```python
from build123d import *

# Parameters (mm, degrees)
F0_R     = 2.15
F1_DEPTH = 250


# Not quite as in the source:
# - ends of sketch curves that miss each other by under 0.0002 mm in the source are joined


with BuildPart() as f1:
    # F0 (on Top) → F1 (new body)
    with BuildSketch(Plane.XY):
        with BuildLine():
            Line((10, 3.5), (10, 9))
            ThreePointArc((10, 9), (9.7071067812, 9.7071067812), (9, 10))
            Line((9, 10), (3.5, 10))
            ThreePointArc((3.5, 10), (2.7928932188, 9.7071067812), (2.5, 9))
            Line((2.5, 9), (2.5, 8.2))
            Line((2.5, 8.2), (4.9, 8.2))
            ThreePointArc((4.9, 8.2), (5.8238795325, 7.5826834324), (5.6071067812, 6.4928932188))
            Line((5.6071067812, 6.4928932188), (3.057107, 3.942893))
            ThreePointArc((3.057107, 3.942893), (2.7326834324, 3.7261204675), (2.35, 3.65))
            Line((2.35, 3.65), (-2.35, 3.65))
            ThreePointArc((-2.35, 3.65), (-2.7326834324, 3.7261204675), (-3.0571067812, 3.9428932188))
            Line((-3.0571067812, 3.9428932188), (-5.607107, 6.492893))
            ThreePointArc((-5.607107, 6.492893), (-5.8238795325, 7.5826834324), (-4.9, 8.2))
            Line((-4.9, 8.2), (-2.5, 8.2))
            Line((-2.5, 8.2), (-2.5, 9))
            ThreePointArc((-2.5, 9), (-2.7928932188, 9.7071067812), (-3.5, 10))
            Line((-3.5, 10), (-9, 10))
            ThreePointArc((-9, 10), (-9.7071067812, 9.7071067812), (-10, 9))
            Line((-10, 9), (-10, 3.5))
            ThreePointArc((-10, 3.5), (-9.7071067812, 2.7928932188), (-9, 2.5))
            Line((-9, 2.5), (-8.2, 2.5))
            Line((-8.2, 2.5), (-8.2, 4.9))
            ThreePointArc((-8.2, 4.9), (-7.5826834324, 5.8238795325), (-6.4928932188, 5.6071067812))
            Line((-6.4928932188, 5.6071067812), (-3.942893, 3.057107))
            ThreePointArc((-3.942893, 3.057107), (-3.7261204675, 2.7326834324), (-3.65, 2.35))
            Line((-3.65, 2.35), (-3.65, -2.35))
            ThreePointArc((-3.65, -2.35), (-3.7261204675, -2.7326834324), (-3.9428932188, -3.0571067812))
            Line((-3.9428932188, -3.0571067812), (-6.492893, -5.607107))
            ThreePointArc((-6.492893, -5.607107), (-7.5826834324, -5.8238795325), (-8.2, -4.9))
            Line((-8.2, -4.9), (-8.2, -2.5))
            Line((-8.2, -2.5), (-9, -2.5))
            ThreePointArc((-9, -2.5), (-9.7071067812, -2.7928932188), (-10, -3.5))
            Line((-10, -3.5), (-10, -9))
            ThreePointArc((-10, -9), (-9.7071067812, -9.7071067812), (-9, -10))
            Line((-9, -10), (-3.5, -10))
            ThreePointArc((-3.5, -10), (-2.7928932188, -9.7071067812), (-2.5, -9))
            Line((-2.5, -9), (-2.5, -8.2))
            Line((-2.5, -8.2), (-4.9, -8.2))
            ThreePointArc((-4.9, -8.2), (-5.8238795325, -7.5826834324), (-5.6071067812, -6.4928932188))
            Line((-5.6071067812, -6.4928932188), (-3.057107, -3.942893))
            ThreePointArc((-3.057107, -3.942893), (-2.7326834324, -3.7261204675), (-2.35, -3.65))
            Line((-2.35, -3.65), (2.35, -3.65))
            ThreePointArc((2.35, -3.65), (2.7326834324, -3.7261204675), (3.0571067812, -3.9428932188))
            Line((3.0571067812, -3.9428932188), (5.607107, -6.492893))
            ThreePointArc((5.607107, -6.492893), (5.8238795325, -7.5826834324), (4.9, -8.2))
            Line((4.9, -8.2), (2.5, -8.2))
            Line((2.5, -8.2), (2.5, -9))
            ThreePointArc((2.5, -9), (2.7928932188, -9.7071067812), (3.5, -10))
            Line((3.5, -10), (9, -10))
            ThreePointArc((9, -10), (9.7071067812, -9.7071067812), (10, -9))
            Line((10, -9), (10, -3.5))
            ThreePointArc((10, -3.5), (9.7071067812, -2.7928932188), (9, -2.5))
            Line((9, -2.5), (8.2, -2.5))
            Line((8.2, -2.5), (8.2, -4.9))
            ThreePointArc((8.2, -4.9), (7.5826834324, -5.8238795325), (6.4928932188, -5.6071067812))
            Line((6.4928932188, -5.6071067812), (3.942893, -3.057107))
            ThreePointArc((3.942893, -3.057107), (3.7261204675, -2.7326834324), (3.65, -2.35))
            Line((3.65, -2.35), (3.65, 2.35))
            ThreePointArc((3.65, 2.35), (3.7261204675, 2.7326834324), (3.9428932188, 3.0571067812))
            Line((3.9428932188, 3.0571067812), (6.492893, 5.607107))
            ThreePointArc((6.492893, 5.607107), (7.5826834324, 5.8238795325), (8.2, 4.9))
            Line((8.2, 4.9), (8.2, 2.5))
            Line((8.2, 2.5), (9, 2.5))
            ThreePointArc((9, 2.5), (9.7071067812, 2.7928932188), (10, 3.5))
        make_face()
        Circle(F0_R, mode=Mode.SUBTRACT)
    extrude(amount=F1_DEPTH)


solid = f1.part
```
Work out the finished part from the listing and answer in its coordinate system (mm). A direction names the side the tool comes from. Give positions to 0.01 mm unless a question says otherwise; leave off trailing zeros. Order: outer loops, then holes, each group sorted by start corner. A loop starts at its lowest first (then second) coordinate and runs counter-clockwise, first axis right, second up. Notation, with made-up numbers: M 72.25,65 L 92.25,65 A17 ccw 92.25,69 Z; hole C -5,-16.75 d11. An arc over 180 degrees is marked long. Return JSON: item names as keys, results as strings.
1) Section A-A, the plane y = 0 is taken. Write down the section's boundary in (x, z).
Resolved:
{"outline": "M -3.65,0 L -2.15,0 L -2.15,250 L -3.65,250 Z; M 2.15,0 L 3.65,0 L 3.65,250 L 2.15,250 Z"}
2) Each of these flat-tipped pins is pushed along its axis until it touches: pin 1 (2.5 mm diameter, centred on x = -1, z = 168.5, fed in from -Y); pin 2 (2.5 mm diameter, centred on x = 0, z = 154, fed in from +Y). Where does it stop, or does it pass through?
Resolved:
{"pin 1": "y = -3.65", "pin 2": "y = 3.65"}
3) A tool of negligible diameter and unlimited length cuts with its end or side. For faces 1 (the flat face through (0, 3.65, 123)), 2 (the flat face through (-2.4, 0.1, 0)), from which of +Z, -Z, +X, -X, +Y, -Y can it reach the whole face along a straight path? Write none if from no direction.
Resolved:
{"face 1": "+Z, -Z, +Y", "face 2": "-Z, +X, -X, +Y, -Y"}
4) Straight lines are drawn through the part: line 1 along Y through (x, z) = (-7.5, 103); line 2 along Y through (x, z) = (0, 76.5); line 3 along X through (y, z) = (-4, 189.5). For each, find the intervals that lie inside material, in ascending order. Write a range as [from, to].
Resolved:
{"line 1": "[-10, -5.85], [5.85, 10]", "line 2": "[-3.65, -2.15], [2.15, 3.65]", "line 3": "[-10, -8.2], [-4.89, -3.11], [3.11, 4.89], [8.2, 10]"}
5) For a pull along X with two mould halves and no side action, classify faces 3 (the flat face through (3.65, 0, 123)), 4 (the flat face through (0, -3.65, 123)), 5 (the flat face through (6, -10, 123)), 6 (the flat face through (-3.65, 0, 123)) as +X half, -X half, draft (parallel to the pull), parting line (faces both ways), or undercut.
Resolved:
{"face 3": "+X half", "face 4": "undercut", "face 5": "draft", "face 6": "-X half"}
